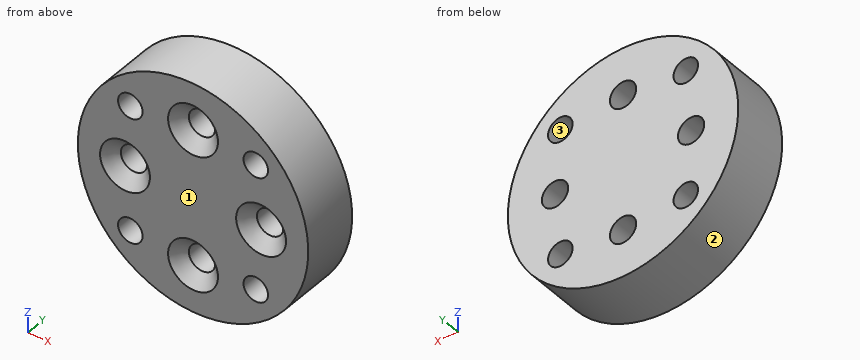
from build123d import *

# Parameters (mm, degrees)
SKETCH2_R                                         = 12.7
BOSS_EXTRUDE1_DEPTH                               = 6.35
CSK_FOR_M2_5_FLAT_HEAD_MACHINE_SCREW1_D           = 2.9
CSK_FOR_M2_5_FLAT_HEAD_MACHINE_SCREW1_CSINK_D     = 5.5
CSK_FOR_M2_5_FLAT_HEAD_MACHINE_SCREW1_CSINK_ANGLE = 90
F_6_32_TAPPED_HOLE1_D                             = 2.7051
F_6_32_TAPPED_HOLE1_DEPTH                         = 9.38784
F_6_32_TAPPED_HOLE1_TIP                           = 0.81269403


with BuildPart() as part:
    # Sketch2 → Boss-Extrude1 (new body)
    with BuildSketch(Plane(origin=(0, 0, 0), x_dir=(1, 0, 0), z_dir=(0, 1, 0))):
        with Locations(Location((0, 0, 0), (0, 0, 270))):
            Circle(SKETCH2_R)
    extrude(amount=BOSS_EXTRUDE1_DEPTH)

    # CSK for M2.5 Flat Head Machine Screw1 (through all)
    with Locations(Plane(origin=(0, 0, 0), x_dir=(-1, 0, 0), z_dir=(0, -1, 0))):
        with Locations((7.5, 0), (-7.5, 0), (0, -7.5), (0, 7.5)):
            CounterSinkHole(CSK_FOR_M2_5_FLAT_HEAD_MACHINE_SCREW1_D / 2, CSK_FOR_M2_5_FLAT_HEAD_MACHINE_SCREW1_CSINK_D / 2, counter_sink_angle=CSK_FOR_M2_5_FLAT_HEAD_MACHINE_SCREW1_CSINK_ANGLE)

    # #6-32 Tapped Hole1
    with Locations(Plane(origin=(0, 0, 0), x_dir=(-1, 0, 0), z_dir=(0, -1, 0))):
        with Locations((6.914797213, -6.914797213), (-6.914797213, -6.914797213), (-6.914797213, 6.914797213), (6.914797213, 6.914797213)):
            Hole(F_6_32_TAPPED_HOLE1_D / 2, depth=F_6_32_TAPPED_HOLE1_DEPTH)
            with Locations((0, 0, -(F_6_32_TAPPED_HOLE1_DEPTH + F_6_32_TAPPED_HOLE1_TIP / 2))):  # 118° drill point
                Cone(0, F_6_32_TAPPED_HOLE1_D / 2, F_6_32_TAPPED_HOLE1_TIP, mode=Mode.SUBTRACT)


solid = part.part
Input: part model. Units: mm. Frame: model coordinates. Face numbers are marked on the shaded views. Coordinates: 2 decimals unless noted, no trailing zeros. Order: outer loops, then holes, each group sorted by start corner. A loop starts at its lowest first (then second) coordinate and runs counter-clockwise, first axis right, second up. Notation, with made-up numbers: M 81,21 L 93,21 A21 cw 93,32 Z; hole C 86,-27 d7. An arc over 180 degrees is marked long. Write item = value, one per line. Start each with the question number.
(1) Section A-A on z = 0. Output: boundary loops of the cut face in (x, y).
(2) Line query: line 1 along X through (y, z) = (4.75, -0.75); line 2 along Z through (x, y) = (7.5, 3.5); line 3 along Z through (x, y) = (1, 4.25). Output: solid intervals per line, ascending. Write a range as [from, to].
(3) Section C-C on x = 7.5. Output: boundary loops of the cut face in (y, z), and give its area (3 significant figures).
(4) First-contact query: P1, Ø4, axis at x = 7.5, z = 0, coming from the -Y side; P2, Ø2, axis at x = -6.91, z = 6.91, coming from the +Y side; P3, Ø1, axis at y = 3, z = 1, coming from the +X side; P4, Ø4.5, axis at x = 0, z = -7.5, coming from the -Y side. Flat tips, straight axial feed; report the tip coordinate or a pass-through.
(5) Section B-B on y = 3. Give the number of separate pieces and of enclosed holes in the cut face, and give its area (3 significant figures).
(6) Pull-direction query (Z, two-part tool) for the marked faces 1, 2 and 3; classes: released by +Z, released by -Z, zero draft, split by the parting line, or undercut.
(7) Section D-D on z = -7.5. Output: boundary loops of the cut face in (x, y).
Result set:
q1.outline = M -12.7,0 L -10.25,0 L -8.95,1.3 L -8.95,6.35 L -12.7,6.35 Z; M -6.05,1.3 L -4.75,0 L 4.75,0 L 6.05,1.3 L 6.05,6.35 L -6.05,6.35 Z; M 8.95,1.3 L 10.25,0 L 12.7,0 L 12.7,6.35 L 8.95,6.35 Z
q2.line_1 = [-12.68, -8.74], [-6.26, 6.26], [8.74, 12.68]
q2.line_2 = [-10.25, -8.13], [-5.7, -1.45], [1.45, 5.7], [8.13, 10.25]
q2.line_3 = [-12.66, -8.55], [-6.45, 6.45], [8.55, 12.66]
q3.outline = M 0,-10.25 L 6.35,-10.25 L 6.35,-8.13 L 0,-8.13 Z; M 0,-5.7 L 6.35,-5.7 L 6.35,-1.45 L 1.3,-1.45 L 0,-2.75 Z; M 0,2.75 L 1.3,1.45 L 6.35,1.45 L 6.35,5.7 L 0,5.7 Z; M 0,8.13 L 6.35,8.13 L 6.35,10.25 L 0,10.25 Z
q3.area = 79.1 mm²
q4.P1 = 0.75
q4.P2 = through
q4.P3 = 12.69
q4.P4 = 0.5
q5.separate_pieces = 1
q5.enclosed_holes = 8
q5.area = 457 mm²
q6.face_1 = zero draft
q6.face_2 = split by the parting line
q6.face_3 = undercut
q7.outline = M -10.25,0 L -8.13,0 L -8.13,6.35 L -10.25,6.35 Z; M -5.7,0 L -2.75,0 L -1.45,1.3 L -1.45,6.35 L -5.7,6.35 Z; M 1.45,1.3 L 2.75,0 L 5.7,0 L 5.7,6.35 L 1.45,6.35 Z; M 8.13,0 L 10.25,0 L 10.25,6.35 L 8.13,6.35 Z
